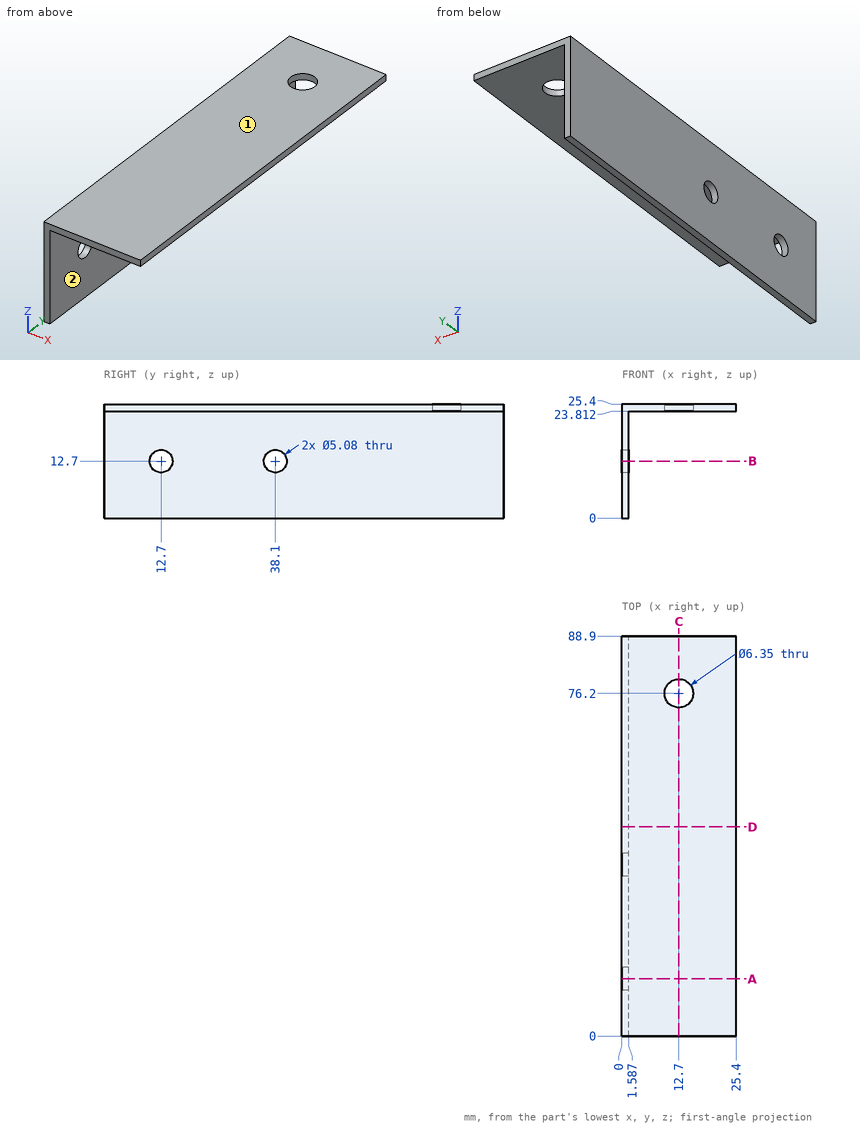
Here's the drawing with two shaded views (mm, measured from the low corner). I have some questions. A direction names the side the tool comes from. Coordinates: 2 decimals unless noted, no trailing zeros. Loops run counter-clockwise (first coordinate to the right, second up) from the corner with the lowest first, then second, coordinate; pieces in that order, holes last. Notation, with made-up numbers: (57.5, 1.5) -> (102.5, 1.5) arc R7 ccw to (102.5, 13.5) -> close; hole circle Ø4 at (65.25, 55). An arc over 180 degrees is marked (long way). Put each result on its own line as item: value. Start each with the question number.
Q1. For the marked faces 1 and 2, which set-ups out of +Z, -Z, +X, -X, +Y, -Y let a thin tool reach every point of the face, with its end or its side?
Q2. I want a section at A-A (y = 12.7). Write out the boundary of the cut face in (x, z).
Q3. I want a section at B-B (z = 12.7). Write out the boundary of the cut face in (x, y), plus the area to 3 significant figures.
Q4. I'm going to push flat-ended pins straight in: P1, Ø5, axis at x = 3.5, z = 16.5, coming from the +Y side; P2, Ø4, axis at y = 49, z = 14, coming from the +X side; P3, Ø6, axis at x = 10.5, y = 62.5, coming from the -Z side. Where does each tip first touch, or does it pass through?
Q5. I want a section at C-C (x = 12.7). Write out the boundary of the cut face in (y, z) (1 decimal).
Q6. I want a section at D-D (y = 46.5). Write out the boundary of the cut face in (x, z).
Q7. If I drill on line 1 (Y direction, x = 0.4, z = 12.7); line 2 (Y direction, x = 12.7, z = 25.15) (1 decimal); line 3 (Z direction, x = 20.75, y = 77), over which ranges is the centre line in solid material (lowest first)? Write a range as [from, to].
Taken from the geometry:
1. face 1: +Z, +X, -X, +Y, -Y
1. face 2: -Z, +X, +Y, -Y
2. outline: (0, 0) -> (1.59, 0) -> (1.59, 10.16) -> (0, 10.16) -> close; (0, 15.24) -> (1.59, 15.24) -> (1.59, 23.81) -> (25.4, 23.81) -> (25.4, 25.4) -> (0, 25.4) -> close
3. outline: (0, 0) -> (1.59, 0) -> (1.59, 10.16) -> (0, 10.16) -> close; (0, 15.24) -> (1.59, 15.24) -> (1.59, 35.56) -> (0, 35.56) -> close; (0, 40.64) -> (1.59, 40.64) -> (1.59, 88.9) -> (0, 88.9) -> close
3. area: 125 mm2
4. P1: stops at y = 88.9
4. P2: stops at x = 1.59
4. P3: stops at z = 23.81
5. outline: (0, 23.8) -> (73, 23.8) -> (73, 25.4) -> (0, 25.4) -> close; (79.4, 23.8) -> (88.9, 23.8) -> (88.9, 25.4) -> (79.4, 25.4) -> close
6. outline: (0, 0) -> (1.59, 0) -> (1.59, 23.81) -> (25.4, 23.81) -> (25.4, 25.4) -> (0, 25.4) -> close
7. line 1: y = [0, 10.16], [15.24, 35.56], [40.64, 88.9]
7. line 2: y = [0, 73], [79.4, 88.9]
7. line 3: z = [23.81, 25.4]
